from build123d import *

# Parameters (mm, degrees)
SKETCH1_W           = 152.4
SKETCH1_H           = 12.7
BOSS_EXTRUDE1_DEPTH = 76.2
SKETCH2_R           = 3.4925
BOSS_EXTRUDE4_DEPTH = 6.35
BOSS_EXTRUDE5_DEPTH = 12.7
CUT_EXTRUDE1_REACH  = 148.188
SKETCH4_R           = 5.3975
SKETCH5_R           = 3.4925
CUT_EXTRUDE2_DEPTH  = 145.941445074


with BuildPart() as part:
    # Sketch1 → Boss-Extrude1 (new body)
    with BuildSketch(Plane(origin=(0, 0, 0), x_dir=(1, 0, 0), z_dir=(0, 1, 0))):
        Rectangle(SKETCH1_W, SKETCH1_H)
    extrude(amount=BOSS_EXTRUDE1_DEPTH)

    # Sketch2 → Boss-Extrude4 (add)
    with BuildSketch(Plane(origin=(0, 0, 0), x_dir=(1, 0, 0), z_dir=(0, 1, 0))):
        Polygon((-76.2, 19.05), (-76.2, 6.35), (76.2, 6.35), (76.2, 31.75), (-76.2, 31.75), align=None)
        with Locations(Location((-63.5, 19.05, 0), (0, 0, 270))):
            Circle(SKETCH2_R, mode=Mode.SUBTRACT)
        with Locations(Location((-38.1, 19.05, 0), (0, 0, 270))):
            Circle(SKETCH2_R, mode=Mode.SUBTRACT)
        with Locations(Location((-12.7, 19.05, 0), (0, 0, 270))):
            Circle(SKETCH2_R, mode=Mode.SUBTRACT)
        with Locations(Location((12.7, 19.05, 0), (0, 0, 270))):
            Circle(SKETCH2_R, mode=Mode.SUBTRACT)
        with Locations(Location((38.1, 19.05, 0), (0, 0, 270))):
            Circle(SKETCH2_R, mode=Mode.SUBTRACT)
        with Locations(Location((63.5, 19.05, 0), (0, 0, 270))):
            Circle(SKETCH2_R, mode=Mode.SUBTRACT)
    extrude(amount=BOSS_EXTRUDE4_DEPTH)

    # Sketch3 → Boss-Extrude5 (add)
    with BuildSketch(Plane.XY.offset(6.35)):
        Polygon((-76.2, 76.2), (-76.2, 120.65), (76.2, 120.65), (76.2, 76.2), (73.025, 76.2), (73.025, 117.475), (-73.025, 117.475), (-73.025, 76.2), align=None)
    extrude(amount=-BOSS_EXTRUDE5_DEPTH)

    # Sketch4 → Cut-Extrude1 (cut, up to next)
    with BuildSketch(Plane(origin=(0, 120.65, 0), x_dir=(1, 0, 0), z_dir=(0, 1, 0)), mode=Mode.PRIVATE) as cut_extrude1_sk1:
        with Locations(Location((-63.5, 0, 0), (0, 0, 270))):
            Circle(SKETCH4_R)
    cut_extrude1_tool1 = extrude(cut_extrude1_sk1.sketch, amount=-CUT_EXTRUDE1_REACH, mode=Mode.PRIVATE) & part.part
    # Sketch4 → Cut-Extrude1 (cut, up to next)
    with BuildSketch(Plane(origin=(0, 120.65, 0), x_dir=(1, 0, 0), z_dir=(0, 1, 0)), mode=Mode.PRIVATE) as cut_extrude1_sk2:
        with Locations(Location((-45.72, 0, 0), (0, 0, 270))):
            Circle(SKETCH4_R)
    cut_extrude1_tool2 = extrude(cut_extrude1_sk2.sketch, amount=-CUT_EXTRUDE1_REACH, mode=Mode.PRIVATE) & part.part
    # Sketch4 → Cut-Extrude1 (cut, up to next)
    with BuildSketch(Plane(origin=(0, 120.65, 0), x_dir=(1, 0, 0), z_dir=(0, 1, 0)), mode=Mode.PRIVATE) as cut_extrude1_sk3:
        with Locations(Location((-27.94, 0, 0), (0, 0, 270))):
            Circle(SKETCH4_R)
    cut_extrude1_tool3 = extrude(cut_extrude1_sk3.sketch, amount=-CUT_EXTRUDE1_REACH, mode=Mode.PRIVATE) & part.part
    # Sketch4 → Cut-Extrude1 (cut, up to next)
    with BuildSketch(Plane(origin=(0, 120.65, 0), x_dir=(1, 0, 0), z_dir=(0, 1, 0)), mode=Mode.PRIVATE) as cut_extrude1_sk4:
        with Locations(Location((-10.16, 0, 0), (0, 0, 270))):
            Circle(SKETCH4_R)
    cut_extrude1_tool4 = extrude(cut_extrude1_sk4.sketch, amount=-CUT_EXTRUDE1_REACH, mode=Mode.PRIVATE) & part.part
    # Sketch4 → Cut-Extrude1 (cut, up to next)
    with BuildSketch(Plane(origin=(0, 120.65, 0), x_dir=(1, 0, 0), z_dir=(0, 1, 0)), mode=Mode.PRIVATE) as cut_extrude1_sk5:
        with Locations(Location((7.62, 0, 0), (0, 0, 270))):
            Circle(SKETCH4_R)
    cut_extrude1_tool5 = extrude(cut_extrude1_sk5.sketch, amount=-CUT_EXTRUDE1_REACH, mode=Mode.PRIVATE) & part.part
    # Sketch4 → Cut-Extrude1 (cut, up to next)
    with BuildSketch(Plane(origin=(0, 120.65, 0), x_dir=(1, 0, 0), z_dir=(0, 1, 0)), mode=Mode.PRIVATE) as cut_extrude1_sk6:
        with Locations(Location((25.4, 0, 0), (0, 0, 270))):
            Circle(SKETCH4_R)
    cut_extrude1_tool6 = extrude(cut_extrude1_sk6.sketch, amount=-CUT_EXTRUDE1_REACH, mode=Mode.PRIVATE) & part.part
    # Sketch4 → Cut-Extrude1 (cut, up to next)
    with BuildSketch(Plane(origin=(0, 120.65, 0), x_dir=(1, 0, 0), z_dir=(0, 1, 0)), mode=Mode.PRIVATE) as cut_extrude1_sk7:
        with Locations(Location((43.18, 0, 0), (0, 0, 270))):
            Circle(SKETCH4_R)
    cut_extrude1_tool7 = extrude(cut_extrude1_sk7.sketch, amount=-CUT_EXTRUDE1_REACH, mode=Mode.PRIVATE) & part.part
    # Sketch4 → Cut-Extrude1 (cut, up to next)
    with BuildSketch(Plane(origin=(0, 120.65, 0), x_dir=(1, 0, 0), z_dir=(0, 1, 0)), mode=Mode.PRIVATE) as cut_extrude1_sk8:
        with Locations(Location((60.96, 0, 0), (0, 0, 270))):
            Circle(SKETCH4_R)
    cut_extrude1_tool8 = extrude(cut_extrude1_sk8.sketch, amount=-CUT_EXTRUDE1_REACH, mode=Mode.PRIVATE) & part.part
    add(cut_extrude1_tool1.solids().sort_by_distance((-63.5, 120.65, 0))[0], mode=Mode.SUBTRACT)
    add(cut_extrude1_tool2.solids().sort_by_distance((-45.72, 120.65, 0))[0], mode=Mode.SUBTRACT)
    add(cut_extrude1_tool3.solids().sort_by_distance((-27.94, 120.65, 0))[0], mode=Mode.SUBTRACT)
    add(cut_extrude1_tool4.solids().sort_by_distance((-10.16, 120.65, 0))[0], mode=Mode.SUBTRACT)
    add(cut_extrude1_tool5.solids().sort_by_distance((7.62, 120.65, 0))[0], mode=Mode.SUBTRACT)
    add(cut_extrude1_tool6.solids().sort_by_distance((25.4, 120.65, 0))[0], mode=Mode.SUBTRACT)
    add(cut_extrude1_tool7.solids().sort_by_distance((43.18, 120.65, 0))[0], mode=Mode.SUBTRACT)
    add(cut_extrude1_tool8.solids().sort_by_distance((60.96, 120.65, 0))[0], mode=Mode.SUBTRACT)

    # Sketch5 → Cut-Extrude2 (cut, through all)
    with BuildSketch(Plane(origin=(0, 0, -6.35), x_dir=(-1, 0, 0), z_dir=(0, 0, -1))):
        with Locations((-57.15, 25.4)):
            Circle(SKETCH5_R)
        with Locations((-19.05, 25.4)):
            Circle(SKETCH5_R)
        with Locations((19.05, 25.4)):
            Circle(SKETCH5_R)
        with Locations((57.15, 25.4)):
            Circle(SKETCH5_R)
    extrude(amount=-CUT_EXTRUDE2_DEPTH, mode=Mode.SUBTRACT)


solid = part.part
Here's how the part is built. I have some questions about the finished solid (model axes, mm). A direction names the side the tool comes from. Coordinates: 2 decimals unless noted, no trailing zeros. Write each loop counter-clockwise with the first axis right and the second up, starting at its lowest first coordinate (ties: lowest second). Pieces come first, ordered by that corner, then holes.
Item 1: If we mould it in two halves opening along Y, with no side actions, what happens to faces 4 (the cylindrical face through (-18.29, 21.99, -0.09)), 5 (the flat face through (-1, 0, -13)), 6 (the cylindrical face through (-54.38, 23.27, -0.09)), 7 (the flat face through (1, 39, -6.35))? For each: +Y half, -Y half, draft (parallel to the pull), parting line (faces both ways), or undercut.
Item 2: I want a section at C-C on z = -20.5. Write out the boundary of the cut face in (x, y), and give its area (3 significant figures).
Item 3: I want a section at A-A on x = -38.1. Count the separate pieces of the cut face and the enclosed holes in it, and give its area (4 significant figures).
Item 4: I want a section at B-B on y = 111.5. Write out the boundary of the cut face in (x, z) (3 decimals), and give its area (3 significant figures).
Item 5: Will these pins go through, and if not, where does the flat tip stop? pin 1 (8 mm diameter, centred on x = -12.7, z = -19.05, fed in from -Y); pin 2 (2 mm diameter, centred on x = -0.5, z = -27.5, fed in from +Y); pin 3 (6 mm diameter, centred on x = -30, y = 78.5, fed in from -Z); pin 4 (8.5 mm diameter, centred on x = 60.96, z = 0, fed in from +Y).
Item 6: On a 3-axis mill with a long thin cutter (end or side, diameter ignored), from which of +Z, -Z, +X, -X, +Y, -Y can I reach the whole of each face in a straight line? I mean faces 1 (the flat face through (-1, 6.35, -19)), 2 (the cylindrical face through (20.61, 119.08, 2.49)), 3 (the flat face through (-1, 76.2, 0)). Say none if no direction works.
Item 7: If I drill on line 1 (Y direction, x = -57, z = -2) (3 decimals); line 2 (X direction, y = 24, z = -2); line 3 (X direction, y = 84, z = 2) (3 decimals), over which ranges is the centre line in solid material (lowest first)?
Findings below:
1. face 4: undercut
1. face 5: -Y half
1. face 6: undercut
1. face 7: draft
2. outline: (-76.2, 0) - (-66.68, 0) - (-66.68, 6.35) - (-76.2, 6.35) - close; (-60.32, 0) - (-41.28, 0) - (-41.28, 6.35) - (-60.32, 6.35) - close; (-34.92, 0) - (-15.88, 0) - (-15.88, 6.35) - (-34.92, 6.35) - close; (-9.52, 0) - (9.52, 0) - (9.52, 6.35) - (-9.52, 6.35) - close; (15.88, 0) - (34.92, 0) - (34.92, 6.35) - (15.88, 6.35) - close; (41.28, 0) - (60.32, 0) - (60.32, 6.35) - (41.28, 6.35) - close; (66.68, 0) - (76.2, 0) - (76.2, 6.35) - (66.68, 6.35) - close
2. area: 726 mm2
3. separate pieces: 3
3. enclosed holes: 0
3. area: 1,125 mm2
4. outline: (-76.2, -6.35) - (-73.025, -6.35) - (-73.025, 6.35) - (-76.2, 6.35) - close; (73.025, -6.35) - (76.2, -6.35) - (76.2, 6.35) - (73.025, 6.35) - close
4. area: 80.6 mm2
5. pin 1: stops at y = 0
5. pin 2: stops at y = 6.35
5. pin 3: stops at z = -6.35
5. pin 4: stops at y = 76.2
6. face 1: -Z, +X, -X, +Y
6. face 2: +Y
6. face 3: +Z, -Z
7. line 1: y = 0 to 21.911, 28.889 to 76.2, 117.475 to 120.65
7. line 2: x = -76.2 to -60.35, -53.95 to -22.25, -15.85 to 15.85, 22.25 to 53.95, 60.35 to 76.2
7. line 3: x = -76.2 to -73.025, 73.025 to 76.2
